Model file for the job. Use its own axes, mm. A direction names the side the tool comes from. Give positions to 0.01 mm unless a question says otherwise; leave off trailing zeros. Write each loop counter-clockwise with the first axis right and the second up, starting at its lowest first coordinate (ties: lowest second). Pieces come first, ordered by that corner, then holes. Notation, with made-up numbers: (49, -14) - (107, -14) arc R24 cw to (107, 4) - close; hole circle Ø3 at (3.5, 28). An arc over 180 degrees is marked (long way). Use CSV: the item, a comma, the result in double quotes.
from build123d import *

# Parameters (mm, degrees)
SKETCH_1_R          = 2.95
EXTRUDE_1_DEPTH     = 2.7
SKETCH_2_R          = 1.5
EXTRUDE_2_DEPTH     = 30
SKETCH_3_R          = 1.25
EXTRUDE_3_DEPTH     = 5
CUT_EXTRUDE_1_DEPTH = 2
FILLET_1_R          = 0.2


with BuildPart() as part:
    # 草图1 → 凸台-拉伸1 (new body)
    with BuildSketch(Plane(origin=(0, 0, 0), x_dir=(1, 0, 0), z_dir=(0, 1, 0))):
        Circle(SKETCH_1_R)
    extrude(amount=EXTRUDE_1_DEPTH)

    # 草图2 → 凸台-拉伸2 (add)
    with BuildSketch(Plane(origin=(0, 2.7, 0), x_dir=(1, 0, 0), z_dir=(0, 1, 0))):
        Circle(SKETCH_2_R)
    extrude(amount=EXTRUDE_2_DEPTH)

    # 草图3 → 凸台-拉伸3 (add)
    with BuildSketch(Plane(origin=(0, 32.7, 0), x_dir=(1, 0, 0), z_dir=(0, 1, 0))):
        Circle(SKETCH_3_R)
    extrude(amount=EXTRUDE_3_DEPTH)

    # 草图4 → 切除-拉伸1 (cut)
    with BuildSketch(Plane.XZ):
        Polygon((2.247285488, -0.53201623), (1.584382314, 1.680198207), (-0.662903174, 2.212214437), (-2.247285488, 0.53201623), (-1.584382314, -1.680198207), (0.662903174, -2.212214437), align=None)
    extrude(amount=-CUT_EXTRUDE_1_DEPTH, mode=Mode.SUBTRACT)

    # 圆角1
    fillet_1_edges = [part.edges().sort_by_distance(p)[0] for p in [
        (-1.25, 37.7, 0),
        (-2.95, 0, 0),
        (-2.95, 2.7, 0),
    ]]
    fillet(fillet_1_edges, radius=FILLET_1_R)


solid = part.part
(1) Saw through at B-B, the plane x = 0. List the corners of the cut face in (y, z).
Checked values:
outline,"(0, -2.75) arc R0.2 ccw to (0.2, -2.95) - (2.5, -2.95) arc R0.2 ccw to (2.7, -2.75) - (2.7, -1.5) - (32.7, -1.5) - (32.7, -1.25) - (37.5, -1.25) arc R0.2 ccw to (37.7, -1.05) - (37.7, 1.05) arc R0.2 ccw to (37.5, 1.25) - (32.7, 1.25) - (32.7, 1.5) - (2.7, 1.5) - (2.7, 2.75) arc R0.2 ccw to (2.5, 2.95) - (0.2, 2.95) arc R0.2 ccw to (0, 2.75) - (0, 2.06) - (2, 2.06) - (2, -2.06) - (0, -2.06) - close"
(2) Wall check: probe 1 along Y at (x, z) = (-0.8, -2.5); probe 2 along Y at (x, z) = (-0.7, 1.8); probe 3 along X at (y, z) = (7.5, 0.05). Give the ranges that are in metal, low to high. Write a range as [from, to].
Checked values:
probe 1,"y = [0, 2.7]"
probe 2,"y = [2, 2.7]"
probe 3,"x = [-1.5, 1.5]"
(3) Pull direction X, two halves, no side cores. Call faces 1 (the face through (1.2, 2.7, 1.2)), 2 (the face through (-1.5, 17.49, -0.07)), 3 (the face through (-1.92, 0.99, -0.56)): released by +X, released by -X, zero draft, split by the parting line, or undercut.
Checked values:
face 1,"zero draft"
face 2,"split by the parting line"
face 3,"undercut"
(4) 3-axis set-ups, long thin cutter, end or side, ignore diameter. For faces 4 (the face through (-0.27, 35.07, 1.22)), 5 (the face through (0, 37.7, 0)), 6 (the face through (0.48, 0.99, 1.94)): which of +Z, -Z, +X, -X, +Y, -Y reach the whole face in a straight line?
Checked values:
face 4,"+Y"
face 5,"+Z, -Z, +X, -X, +Y"
face 6,"-Y"
(5) Saw through at A-A, the plane z = 0. List the corners of the cut face in (x, y).
Checked values:
outline,"(-2.95, 0.2) arc R0.2 ccw to (-2.75, 0) - (-2.09, 0) - (-2.09, 2) - (2.09, 2) - (2.09, 0) - (2.75, 0) arc R0.2 ccw to (2.95, 0.2) - (2.95, 2.5) arc R0.2 ccw to (2.75, 2.7) - (1.5, 2.7) - (1.5, 32.7) - (1.25, 32.7) - (1.25, 37.5) arc R0.2 ccw to (1.05, 37.7) - (-1.05, 37.7) arc R0.2 ccw to (-1.25, 37.5) - (-1.25, 32.7) - (-1.5, 32.7) - (-1.5, 2.7) - (-2.75, 2.7) arc R0.2 ccw to (-2.95, 2.5) - close"
(6) Flat gauge pins, fed straight in: P1, Ø1.5, axis at y = 24.5, z = 0, coming from the -X side; P2, Ø3, axis at x = 0.5, y = 8.5, coming from the +Z side. Where does each tip first touch, or does it go through?
Checked values:
P1,"stops at x = -1.5"
P2,"stops at z = 1.5"
(7) Saw through at C-C, the plane y = 5. List the corners of the cut face in (x, z), then the cut area to 3 significant figures.
Checked values:
outline,"circle Ø3 at (0, 0)"
area,"7.07 mm^2"
